Could you check a few things on this model? Use its own coordinates, in mm. Coordinates: 2 decimals unless noted, no trailing zeros. Loops run counter-clockwise (first coordinate to the right, second up) from the corner with the lowest first, then second, coordinate; pieces in that order, holes last.
1) Imagine slicing it at A-A on z = -1. Please give me the cut outline in (x, y), plus the area to 3 significant figures.
2) Imagine slicing it at B-B on y = 1.5. Please give me the cut outline in (x, z), plus the area to 3 significant figures.
3) Will these pins go through, and if not, where does the flat tip stop? P1, Ø1, axis at y = 2, z = -6, coming from the -X side; P2, Ø1, axis at y = 1.5, z = -8, coming from the +X side; P3, Ø1, axis at x = -10, y = 1, coming from the -Z side; P4, Ø2.5, axis at x = -20, z = 0, coming from the +Y side.
4) Imagine slicing it at C-C on x = -33. Please give me the cut outline in (y, z), plus the area to 3 significant figures.
5) If I drill on line 1 along Z through (x, y) = (0, 1.55); line 2 along X through (y, z) = (1.3, 1.75); line 3 along X through (y, z) = (1.6, -1.75), over which ranges is the centre line in solid material (lowest first)?
6) Imagine slicing it at D-D on z = -10.25. Please give me the cut outline in (x, y).
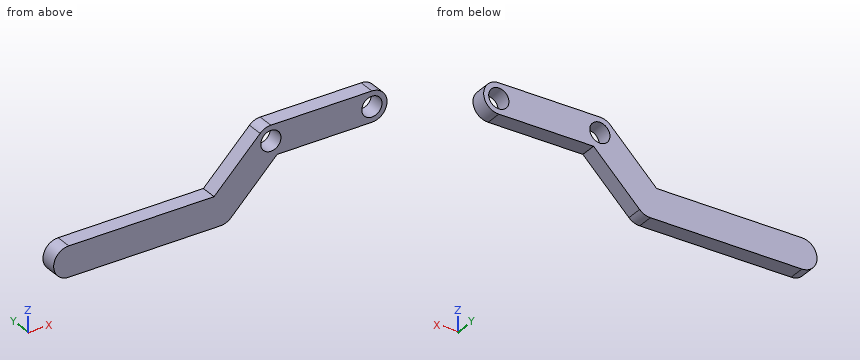
Autodesk Inventor part; units mm, degrees
ref_plane "YZ Plane" through (0, 0, 0) normal (1, 0, 0) x (0, 1, 0)
ref_plane "XZ Plane" through (0, 0, 0) normal (0, 1, 0) x (-1, 0, 0)
ref_plane "XY Plane" through (0, 0, 0) normal (0, 0, 1) x (1, 0, 0)
sketch "Boceto1" plane through (0, 0, 0) normal (0, 1, 0) x (-1, 0, 0)
  circle A0 centre (0, 0) radius 2
  line L0 (0, 0) -> (20, 0) construction
  line L1 (0, -3) -> (20, -3)
  line L2 (20, 3) -> (0, 3)
  arc A1 (0, 3) -> (0, -3) centre (0, 0) ccw
  arc A2 (20, -3) -> (20, 3) centre (20, 0) ccw
  circle A3 centre (20, 0) radius 2
  line L3 (20, 0) -> (30, -10) construction
  line L4 (17.8787, -2.1213) -> (27.8787, -12.1213)
  line L5 (32.1213, -7.8787) -> (22.1213, 2.1213)
  arc A4 (22.1213, 2.1213) -> (17.8787, -2.1213) centre (20, 0) ccw
  arc A5 (27.8787, -12.1213) -> (32.1213, -7.8787) centre (30, -10) ccw
  line L6 (30, -10) -> (60, -10) construction
  line L7 (30, -13) -> (60, -13)
  line L8 (60, -7) -> (30, -7)
  arc A6 (30, -7) -> (30, -13) centre (30, -10) ccw
  arc A7 (60, -13) -> (60, -7) centre (60, -10) ccw
  point P0 (10, 0)
  point P1 (25, -5)
  point P2 (45, -10)
  dimension "d0" = 4
  dimension "d1" = 6
  dimension "d2" = 20
  dimension "d3" = 4
  dimension "d4" = 6
  dimension "d5" = 5
  dimension "d6" = 5
  dimension "d7" = 6
  dimension "d8" = 30
extrude "Extrusión1" add sketch "Boceto1" along normal blind 3.18
properties part number "PINZA_DEDO"
Filled in:
1. outline: (-25.24, 0) - (-21.73, 0) - (-21.73, 3.18) - (-25.24, 3.18) - close; (-18.27, 0) - (-1.73, 0) - (-1.73, 3.18) - (-18.27, 3.18) - close; (1.73, 0) - (2.83, 0) - (2.83, 3.18) - (1.73, 3.18) - close
1. area: 67.2 mm2
2. outline: (-60, -13) - (-30, -13) arc R3 ccw to (-27.88, -12.12) - (-18.76, -3) - (0, -3) arc R3 ccw to (0, 3) - (-20, 3) arc R3 ccw to (-22.12, 2.12) - (-31.24, -7) - (-60, -7) arc R3 ccw to start; hole circle Ø4 at (-20, 0); hole circle Ø4 at (0, 0)
2. area: 388 mm2
3. P1: stops at x = -30.74
3. P2: stops at x = -23.26
3. P3: stops at z = -3
3. P4: passes through
4. outline: (0, -13) - (3.18, -13) - (3.18, -7) - (0, -7) - close
4. area: 19.1 mm2
5. line 1: z = -3 to -2, 2 to 3
5. line 2: x = -22.49 to -20.97, -19.03 to -0.97, 0.97 to 2.44
5. line 3: x = -25.99 to -20.97, -19.03 to -0.97, 0.97 to 2.44
6. outline: (-62.99, 0) - (-26.01, 0) - (-26.01, 3.18) - (-62.99, 3.18) - close
